Autodesk Fusion 360 part; units mm, degrees
sketch "Sketch1" plane through (0, 0, 0) normal (0, 0, 1) x (1, 0, 0)
  line L0 (25, 75) -> (55, 75)
  line L1 (55, 75) -> (55, 45)
  line L2 (55, 45) -> (25, 45)
  line L3 (25, 45) -> (25, 75)
  dimension "d1" = 30
  dimension "d2" = 30
extrude "Extrude1" add sketch "Sketch1" along normal blind 55
sketch "Sketch2" plane through (0, 0, 0) normal (0, 0, 1) x (1, 0, 0)
  line L0 (25, 75) -> (25, 70)
  line L1 (25, 70) -> (50, 70)
  line L2 (50, 70) -> (50, 50)
  line L3 (50, 50) -> (30, 50)
  line L4 (30, 50) -> (30, 70)
  dimension "d5" = 5
  dimension "d6" = 25
  dimension "d7" = 20
  dimension "d8" = 20
extrude "Extrude2" cut sketch "Sketch2" along normal blind 55
sketch "Sketch3" plane through (25, 0, 0) normal (-1, 0, 0) x (0, -1, 0)
  line L0 (-75, 0) -> (-45, 0)
  line L1 (-45, 0) -> (-45, 55)
  line L2 (-45, 55) -> (-75, 55)
  line L3 (-75, 55) -> (-75, 0)
  line L4 (-70, 50) -> (-50, 50)
  line L5 (-50, 50) -> (-50, 30)
  line L6 (-50, 30) -> (-70, 30)
  line L7 (-70, 30) -> (-70, 50)
  line L8 (-70, 25) -> (-50, 25)
  line L9 (-50, 25) -> (-50, 5)
  line L10 (-50, 5) -> (-70, 5)
  line L11 (-70, 5) -> (-70, 25)
extrude "Extrude3" cut sketch "Sketch3" against normal blind 6 contours L4 L5 L6 L7 | L8 L9 L10 L11
sketch "Sketch4" plane through (0, 45, 0) normal (0, -1, 0) x (1, 0, 0)
  line L0 (25, 0) -> (55, 0)
  line L1 (55, 0) -> (55, 55)
  line L2 (55, 55) -> (25, 55)
  line L3 (25, 55) -> (25, 0)
  line L4 (30, 50) -> (50, 50)
  line L5 (50, 50) -> (50, 30)
  line L6 (50, 30) -> (30, 30)
  line L7 (30, 50) -> (30, 30)
  line L8 (30, 25) -> (50, 25)
  line L9 (50, 25) -> (50, 5)
  line L10 (50, 5) -> (30, 5)
  line L11 (30, 5) -> (30, 25)
extrude "Extrude4" cut sketch "Sketch4" against normal blind 5 contours L4 L5 L6 L7 | L8 L9 L10 L11
sketch "Sketch5" plane through (55, 0, 0) normal (1, 0, 0) x (0, 1, 0)
  line L0 (45, 0) -> (75, 0)
  line L1 (75, 0) -> (75, 55)
  line L2 (75, 55) -> (45, 55)
  line L3 (45, 55) -> (45, 0)
  line L4 (50, 50) -> (70, 50)
  line L5 (70, 50) -> (70, 30)
  line L6 (70, 30) -> (50, 30)
  line L7 (50, 30) -> (50, 50)
  line L8 (50, 25) -> (70, 25)
  line L9 (70, 25) -> (70, 5)
  line L10 (70, 5) -> (50, 5)
  line L11 (50, 5) -> (50, 25)
extrude "Extrude5" cut sketch "Sketch5" against normal blind 5 contours L4 L5 L6 L7 | L8 L9 L10 L11
sketch "Sketch6" plane through (0, 0, 0) normal (0, 0, -1) x (1, 0, 0)
  line L0 (30, -70) -> (30, -50)
  line L1 (30, -50) -> (50, -50)
  line L2 (50, -50) -> (50, -70)
  line L3 (50, -70) -> (30, -70)
  line L4 (55, -45) -> (25, -45)
  line L5 (25, -45) -> (25, -75)
  line L6 (25, -75) -> (55, -75)
  line L7 (55, -75) -> (55, -45)
sketch "Sketch7" plane through (55, 0, 0) normal (1, 0, 0) x (0, 1, 0)
  line L0 (70, 50) -> (70, 30)
  line L1 (70, 30) -> (50, 30)
  line L2 (50, 30) -> (50, 50)
  line L3 (50, 50) -> (70, 50)
  line L4 (70, 25) -> (70, 5)
  line L5 (70, 5) -> (50, 5)
  line L6 (50, 5) -> (50, 25)
  line L7 (50, 25) -> (70, 25)
  line L8 (45, 0) -> (75, 0)
  line L9 (75, 0) -> (75, 55)
  line L10 (75, 55) -> (45, 55)
  line L11 (45, 55) -> (45, 0)
  line L12 (75, 0) -> (84, 0)
  line L13 (84, 0) -> (89, 0)
  line L14 (84, 0) -> (84, 55)
  line L15 (84, 55) -> (89, 55)
  line L16 (89, 55) -> (89, 0)
  line L17 (75, 0) -> (75, 5)
  line L18 (75, 5) -> (84, 5)
  dimension "d17" = 9
  dimension "d18" = 5
  dimension "d19" = 5
extrude "Extrude6" add sketch "Sketch7" against normal blind 30 contours L9 L12 L14 L17 L18 | L13 L14 L15 L16
sketch "Sketch8" plane through (0, 0, 0) normal (1, 0, 0) x (0, 1, 0)
sketch "Sketch9" plane through (25, 0, 0) normal (-1, 0, 0) x (0, -1, 0)
  line L0 (-50, 50) -> (-50, 30)
  line L1 (-50, 30) -> (-70, 30)
  line L2 (-70, 30) -> (-70, 50)
  line L3 (-70, 50) -> (-50, 50)
  line L4 (-50, 25) -> (-50, 5)
  line L5 (-50, 5) -> (-70, 5)
  line L6 (-70, 5) -> (-70, 25)
  line L7 (-70, 25) -> (-50, 25)
  line L8 (-89, 0) -> (-45, 0)
  line L9 (-45, 0) -> (-45, 55)
  line L10 (-45, 55) -> (-75, 55)
  line L11 (-75, 55) -> (-75, 5)
  line L12 (-75, 5) -> (-84, 5)
  line L13 (-84, 5) -> (-84, 55)
  line L14 (-84, 55) -> (-89, 55)
  line L15 (-89, 55) -> (-89, 0)
  line L16 (-50, 5) -> (-70, 5)
  line L17 (-70, 5) -> (-70, 25)
  line L18 (-70, 25) -> (-50, 25)
  line L19 (-50, 25) -> (-50, 5)
extrude "Extrude7" add sketch "Sketch9" against normal blind 5 contours L4 L5 L6 L7 L16 L17 L18 L19
sketch "Sketch10" plane through (25, 0, 0) normal (-1, 0, 0) x (0, -1, 0)
  line L0 (-50, 50) -> (-50, 30)
  line L1 (-50, 30) -> (-70, 30)
  line L2 (-70, 30) -> (-70, 50)
  line L3 (-70, 50) -> (-50, 50)
  line L4 (-89, 0) -> (-45, 0)
  line L5 (-45, 0) -> (-45, 55)
  line L6 (-45, 55) -> (-75, 55)
  line L7 (-75, 55) -> (-75, 5)
  line L8 (-75, 5) -> (-84, 5)
  line L9 (-84, 5) -> (-84, 55)
  line L10 (-84, 55) -> (-89, 55)
  line L11 (-89, 55) -> (-89, 0)
  line L12 (-60, 0) -> (-60, 15)
  circle A0 centre (-60, 15) radius 2.5
  dimension "d24" = 5
extrude "Extrude8" cut sketch "Sketch10" against normal blind 5 contours A0
sketch "Sketch11" plane through (55, 0, 0) normal (1, 0, 0) x (0, 1, 0)
  line L0 (70, 50) -> (70, 30)
  line L1 (70, 30) -> (50, 30)
  line L2 (50, 30) -> (50, 50)
  line L3 (50, 50) -> (70, 50)
  line L4 (70, 25) -> (70, 5)
  line L5 (70, 5) -> (50, 5)
  line L6 (50, 5) -> (50, 25)
  line L7 (50, 25) -> (70, 25)
  line L8 (45, 0) -> (89, 0)
  line L9 (89, 0) -> (89, 55)
  line L10 (89, 55) -> (84, 55)
  line L11 (84, 55) -> (84, 5)
  line L12 (84, 5) -> (75, 5)
  line L13 (75, 5) -> (75, 55)
  line L14 (75, 55) -> (45, 55)
  line L15 (45, 55) -> (45, 0)
  line L16 (70, 30) -> (50, 30)
  line L17 (50, 30) -> (50, 50)
  line L18 (50, 50) -> (70, 50)
  line L19 (70, 50) -> (70, 30)
extrude "Extrude9" add sketch "Sketch11" against normal blind 5 contours L0 L1 L2 L3 L16 L17 L18 L19
sketch "Sketch12" plane through (55, 0, 0) normal (1, 0, 0) x (0, 1, 0)
  line L0 (70, 25) -> (70, 5)
  line L1 (70, 5) -> (50, 5)
  line L2 (50, 5) -> (50, 25)
  line L3 (50, 25) -> (70, 25)
  line L4 (45, 0) -> (89, 0)
  line L5 (89, 0) -> (89, 55)
  line L6 (89, 55) -> (84, 55)
  line L7 (84, 55) -> (84, 5)
  line L8 (84, 5) -> (75, 5)
  line L9 (75, 5) -> (75, 55)
  line L10 (75, 55) -> (45, 55)
  line L11 (45, 55) -> (45, 0)
  line L12 (60, 55) -> (60, 40)
  circle A0 centre (60, 40) radius 2.5
  dimension "d29" = 5
extrude "Extrude10" cut sketch "Sketch12" against normal blind 5 contours A0
Input: part model. Units: mm. Frame: model coordinates. A direction names the side the tool comes from. Give positions to 0.01 mm unless a question says otherwise; leave off trailing zeros. Order: outer loops, then holes, each group sorted by start corner. A loop starts at its lowest first (then second) coordinate and runs counter-clockwise, first axis right, second up. Notation, with made-up numbers: M -23,77.5 L -6,77.5 A13 cw -6,94.5 Z; hole C 28,15.5 d9. An arc over 180 degrees is marked long. One line per question, with ' | ' between items. Start each with the question number.
1. Section query C-C (y = 60). Return the cut outline in (x, z).
2. Section query A-A (z = 15). Return the cut outline in (x, y), and give its area (3 significant figures).
3. Pull-direction query (Y, two-part tool) for faces 1 (the face through (53, 60, 25)), 2 (the face through (52.54, 62.31, 39.04)), 3 (the face through (30, 47, 40)), 4 (the face through (40, 45, 27)); classes: released by +Y, released by -Y, zero draft, split by the parting line, or undercut.
4. Material intervals for probe 1 along Y at (x, z) = (26.5, 43); probe 2 along Z at (x, y) = (41.5, 49); probe 3 along Y at (x, z) = (53.4, 40), sorted ascending. Write a range as [from, to].
5. Section query B-B (x = 33.75). Return the cut outline in (y, z).
6. Access query for faces 5 (the face through (40, 50, 53)), 6 (the face through (40, 84, 30)), 7 (the face through (30, 57, 15)). Directions: +Z, -Z, +X, -X, +Y, -Y. A direction counts if a zero-diameter tool reaches every point of the face in a straight line with its end or side. Return the directions, or none.
7. First-contact query: pin 1 Ø4.5 at (x, y) = (38, 78.5) entering from +Z; pin 2 Ø4 at (x, y) = (37.5, 47) entering from -Z; pin 3 Ø3 at (y, z) = (60, 40) entering from +X; pin 4 Ø2 at (x, z) = (34.5, 8.5) entering from -Y. Flat tips, straight axial feed; report the tip coordinate or a pass-through.
8. Section query D-D (z = 32). Return the cut outline in (x, y), and give its area (3 significant figures).
Here are the results:
1) outline: M 25,0 L 30,0 L 30,12.5 L 25,12.5 Z; M 25,17.5 L 30,17.5 L 30,30 L 25,30 Z; M 25,50 L 30,50 L 30,55 L 25,55 Z; M 50,0 L 55,0 L 55,5 L 50,5 Z; M 50,25 L 55,25 L 55,37.5 L 50,37.5 Z; M 50,42.5 L 55,42.5 L 55,55 L 50,55 Z
2) outline: M 25,45 L 30,45 L 30,57.5 L 25,57.5 Z; M 25,62.5 L 30,62.5 L 30,70 L 55,70 L 55,75 L 25,75 Z; M 25,84 L 55,84 L 55,89 L 25,89 Z; M 50,45 L 55,45 L 55,50 L 50,50 Z | area: 425 mm²
3) face 1: undercut | face 2: undercut | face 3: zero draft | face 4: released by -Y
4) probe 1: [45, 50], [70, 75], [84, 89] | probe 2: [0, 5], [25, 30], [50, 55] | probe 3: [45, 57.5], [62.5, 75], [84, 89]
5) outline: M 45,0 L 50,0 L 50,5 L 45,5 Z; M 45,25 L 50,25 L 50,30 L 45,30 Z; M 45,50 L 50,50 L 50,55 L 45,55 Z; M 70,0 L 89,0 L 89,55 L 84,55 L 84,5 L 75,5 L 75,55 L 70,55 Z
6) face 5: +Z, -Z | face 6: +Z, +X, -X | face 7: none
7) pin 1: z = 5 | pin 2: z = 0 | pin 3: through | pin 4: y = 70
8) outline: M 25,45 L 30,45 L 30,50 L 25,50 Z; M 25,70 L 50,70 L 50,45 L 55,45 L 55,75 L 25,75 Z; M 25,84 L 55,84 L 55,89 L 25,89 Z | area: 450 mm²
